Can you work these out from the model? Positions are in its coordinate system, mm. A direction names the side the tool comes from. Coordinates: 2 decimals unless noted, no trailing zeros. Order: outer loops, then holes, each group sorted by start corner. A loop starts at its lowest first (then second) coordinate and runs counter-clockwise, first axis right, second up. Notation, with made-up numbers: (7.25, -4) -> (43.25, -4) arc R21 cw to (43.25, 17) -> close; hole circle Ø8 at (3, -38). An arc over 180 degrees is marked (long way). Write item = value, one per line.
```python
from build123d import *
from OCP.BRepAlgoAPI import BRepAlgoAPI_Cut
from OCP.TopTools import TopTools_ListOfShape

# Parameters (mm, degrees)
CUT_EXTRUDE1_DEPTH      = 10.178779875
CUT_EXTRUDE1_DEPTH_BACK = 10.178779875
CUT_EXTRUDE2_DEPTH      = 2.2
FILLET1_R               = 0.5
CHAMFER1_SIZE           = 1.25
FILLET2_R               = 0.2
CUT_EXTRUDE3_DEPTH      = 9.935323193
CUT_EXTRUDE3_DEPTH_BACK = 9.935323193
SKETCH5_R               = 2.575


with BuildPart() as part:
    # Sketch3 → Revolve1 (revolve)
    with BuildSketch(Plane(origin=(0, 0, 0), x_dir=(0, 0, -1), z_dir=(1, 0, 0)), mode=Mode.PRIVATE) as revolve1_sk:
        Polygon((-1.5, 0), (3.5, 0), (3.5, 6), (1, 6), (-1.5, 6), (-1.5, 3.75), align=None)
    revolve(revolve1_sk.sketch.rotate(Axis((0, 0, 1.5), (0, 0, -1)), 90), axis=Axis((0, 0, 1.5), (0, 0, -1)))

    # Sketch2 → Cut-Extrude1 (cut, two sides: drawn at the far end of the back side and taken through both)
    with BuildSketch(Plane.XY.offset(-CUT_EXTRUDE1_DEPTH_BACK)):
        with BuildLine():
            Line((1.0775, 1.0775), (2.338721606, 1.0775))
            ThreePointArc((2.338721606, 1.0775), (2.575, 0), (2.338721606, -1.0775))
            Line((2.338721606, -1.0775), (1.0775, -1.0775))
            Line((1.0775, -1.0775), (1.0775, -2.338721606))
            ThreePointArc((1.0775, -2.338721606), (0, -2.575), (-1.0775, -2.338721606))
            Line((-1.0775, -2.338721606), (-1.0775, -1.0775))
            Line((-1.0775, -1.0775), (-2.338721606, -1.0775))
            ThreePointArc((-2.338721606, -1.0775), (-2.575, 0), (-2.338721606, 1.0775))
            Line((-2.338721606, 1.0775), (-1.0775, 1.0775))
            Line((-1.0775, 1.0775), (-1.0775, 2.338721606))
            ThreePointArc((-1.0775, 2.338721606), (0, 2.575), (1.0775, 2.338721606))
            Line((1.0775, 2.338721606), (1.0775, 1.0775))
        make_face()
    extrude(amount=CUT_EXTRUDE1_DEPTH + CUT_EXTRUDE1_DEPTH_BACK, mode=Mode.SUBTRACT)

    # Sketch4 → Cut-Extrude2 (cut)
    with BuildSketch(Plane(origin=(0, 0, -3.5), x_dir=(-1, 0, 0), z_dir=(0, 0, -1))):
        with BuildLine():
            Line((-1.5, 4.769696007), (-1.5, 3.096194078))
            Line((-1.5, 3.096194078), (-3.096194078, 1.5))
            Line((-3.096194078, 1.5), (-4.769696007, 1.5))
            ThreePointArc((-4.769696007, 1.5), (-4.942088629, 0.758788496), (-5, 0))
            ThreePointArc((-5, 0), (-4.942088629, -0.758788496), (-4.769696007, -1.5))
            Line((-4.769696007, -1.5), (-3.096194078, -1.5))
            Line((-3.096194078, -1.5), (-1.5, -3.096194078))
            Line((-1.5, -3.096194078), (-1.5, -4.769696007))
            ThreePointArc((-1.5, -4.769696007), (-0.758788496, -4.942088629), (0, -5))
            ThreePointArc((0, -5), (0.758788496, -4.942088629), (1.5, -4.769696007))
            Line((1.5, -4.769696007), (1.5, -3.096194078))
            Line((1.5, -3.096194078), (3.096194078, -1.5))
            Line((3.096194078, -1.5), (4.769696007, -1.5))
            ThreePointArc((4.769696007, -1.5), (4.942088629, -0.758788496), (5, 0))
            ThreePointArc((5, 0), (4.942088629, 0.758788496), (4.769696007, 1.5))
            Line((4.769696007, 1.5), (3.096194078, 1.5))
            Line((3.096194078, 1.5), (1.5, 3.096194078))
            Line((1.5, 3.096194078), (1.5, 4.769696007))
            ThreePointArc((1.5, 4.769696007), (0.758788496, 4.942088629), (0, 5))
            ThreePointArc((0, 5), (-0.758788496, 4.942088629), (-1.5, 4.769696007))
        make_face()
    extrude(amount=-CUT_EXTRUDE2_DEPTH, mode=Mode.SUBTRACT)

    # Fillet1
    fillet1_edges = [part.edges().sort_by_distance(p)[0] for p in [
        (-1.5, 3.096194078, -2.4),
        (-3.096194078, 1.5, -2.4),
        (-3.096194078, -1.5, -2.4),
        (-1.5, -3.096194078, -2.4),
        (1.5, -3.096194078, -2.4),
        (3.096194078, -1.5, -2.4),
        (3.096194078, 1.5, -2.4),
        (1.5, 3.096194078, -2.4),
    ]]
    fillet(fillet1_edges, radius=FILLET1_R)

    # Chamfer1
    chamfer1_edges = [part.edges().sort_by_distance(p)[0] for p in [
        (-6, 0, 1.5),
    ]]
    chamfer(chamfer1_edges, length=CHAMFER1_SIZE)

    # Fillet2
    fillet2_edges = [part.edges().sort_by_distance(p)[0] for p in [
        (2.298097039, -2.298097039, -3.5),
        (-1.5, 4.036498433, -3.5),
        (-2.298097039, 2.298097039, -3.5),
        (-4.036498433, -1.5, -3.5),
        (-2.298097039, -2.298097039, -3.5),
        (1.5, -4.036498433, -3.5),
        (4.036498433, 1.5, -3.5),
        (2.298097039, 2.298097039, -3.5),
        (3.111959143, 1.538060234, -3.5),
        (1.538060234, 3.111959143, -3.5),
        (-1.538060234, 3.111959143, -3.5),
        (-3.111959143, 1.538060234, -3.5),
        (-3.111959143, -1.538060234, -3.5),
        (-1.538060234, -3.111959143, -3.5),
        (1.538060234, -3.111959143, -3.5),
        (3.111959143, -1.538060234, -3.5),
        (-4.75, 0, 1.5),
        (-2.575, 0, 1.5),
        (-1.708110803, -1.0775, 1.5),
        (-1.0775, -1.708110803, 1.5),
        (0, -2.575, 1.5),
        (1.0775, -1.708110803, 1.5),
        (1.708110803, -1.0775, 1.5),
        (2.575, 0, 1.5),
        (1.708110803, 1.0775, 1.5),
        (1.0775, 1.708110803, 1.5),
        (0, 2.575, 1.5),
        (-1.0775, 1.708110803, 1.5),
        (-1.708110803, 1.0775, 1.5),
        (-6, 0, -3.5),
        (0, 5, -3.5),
        (1.5, 4.036498433, -3.5),
        (5, 0, -3.5),
        (4.036498433, -1.5, -3.5),
        (0, -5, -3.5),
        (-1.5, -4.036498433, -3.5),
        (-5, 0, -3.5),
        (-4.036498433, 1.5, -3.5),
    ]]
    fillet(fillet2_edges, radius=FILLET2_R)


with BuildPart() as cut_extrude3_tool:
    # Sketch5 → Cut-Extrude3 (new, two sides: drawn at the far end of the back side and taken through both)
    with BuildSketch(Plane(origin=(0, 0, -1.3), x_dir=(-1, 0, 0), z_dir=(0, 0, -1)).offset(-CUT_EXTRUDE3_DEPTH_BACK)):
        with Locations(Location((0, 0, 0), (0, 0, 155.263446238))):
            Circle(SKETCH5_R)
    extrude(amount=CUT_EXTRUDE3_DEPTH + CUT_EXTRUDE3_DEPTH_BACK)


with BuildPart() as part_1:
    add(part.part)

    # Cut-Extrude3: cut by cut_extrude3_tool, with a tolerance
    cut_extrude3_stock = TopTools_ListOfShape()
    cut_extrude3_stock.Append(part_1.part.wrapped)
    cut_extrude3_tools = TopTools_ListOfShape()
    cut_extrude3_tools.Append(cut_extrude3_tool.part.wrapped)
    cut_extrude3_cut = BRepAlgoAPI_Cut()
    cut_extrude3_cut.SetArguments(cut_extrude3_stock)
    cut_extrude3_cut.SetTools(cut_extrude3_tools)
    cut_extrude3_cut.SetFuzzyValue(0.00001)
    cut_extrude3_cut.Build()
    add(Compound.cast(cut_extrude3_cut.Shape()).solids(), mode=Mode.REPLACE)


solid = part_1.part
```
Item 1: I'm going to push flat-ended pins straight in: P1, Ø1.5, axis at x = -3.5, z = -1, coming from the +Y side; P2, Ø1.6, axis at x = 4, z = -3, coming from the -Y side; P3, Ø1.6, axis at x = -4.5, z = -2.5, coming from the +Y side. Where does each tip first touch, or does it pass through?
A:
P1 = 5.33
P2 = -5.08
P3 = 4.72
Item 2: I want a section at C-C, the plane z = -1.95. Please give me the cut outline in (x, y), plus the area to 3 significant figures.
A:
outline = circle Ø12 at (0, 0); hole (-4.77, -1.5) -> (-3.3, -1.5) arc R0.5 cw to (-2.95, -1.65) -> (-1.65, -2.95) arc R0.5 cw to (-1.5, -3.3) -> (-1.5, -4.77) arc R5 ccw to (1.5, -4.77) -> (1.5, -3.3) arc R0.5 cw to (1.65, -2.95) -> (2.95, -1.65) arc R0.5 cw to (3.3, -1.5) -> (4.77, -1.5) arc R5 ccw to (4.77, 1.5) -> (3.3, 1.5) arc R0.5 cw to (2.95, 1.65) -> (1.65, 2.95) arc R0.5 cw to (1.5, 3.3) -> (1.5, 4.77) arc R5 ccw to (-1.5, 4.77) -> (-1.5, 3.3) arc R0.5 cw to (-1.65, 2.95) -> (-2.95, 1.65) arc R0.5 cw to (-3.3, 1.5) -> (-4.77, 1.5) arc R5 ccw to start
area = 57.9 mm2
Item 3: If we mould it in two halves opening along Y, with no side actions, what happens to faces 1 (the flat face through (2, 2, 1.5)), 2 (the flat face through (-1.5, 4, -2))? For each: pulls with the +Y half, pulls with the -Y half, needs draft (parallel to the pull), parting line crosses it, or undercut.
A:
face_1 = needs draft
face_2 = undercut
Item 4: If I drill on probe 1 along X at (y, z) = (4, -1.6); probe 2 along Z at (x, y) = (2.75, 1.75); probe 3 along X at (y, z) = (2.5, -2.55), over which ranges is the centre line in solid material (lowest first)?
A:
probe_1 = -4.47 to -1.5, 1.5 to 4.47
probe_2 = -1.3 to 1.5
probe_3 = -5.45 to -2.1, 2.1 to 5.45
Item 5: For faces 3 (the cylindrical face through (-2.33, 2.35, -3.44)), 4 (the flat face through (-2.5, -2.7, -3.5)), which set-ups out of +Z, -Z, +X, -X, +Y, -Y let a thin tool reach every point of the face, with its end or its side?
A:
face_3 = -Z
face_4 = -Z, +X, -X, +Y, -Y
